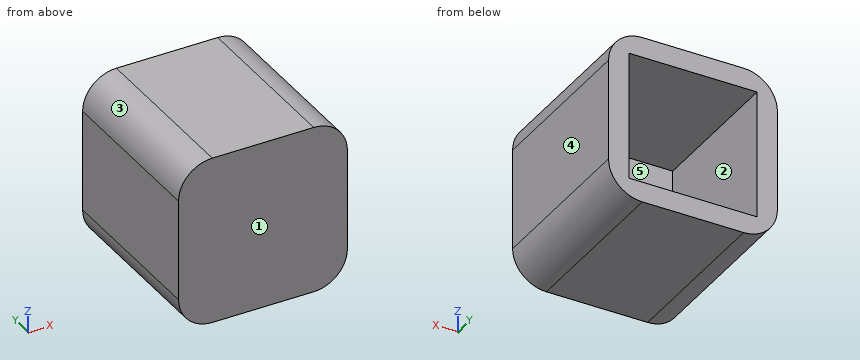
```python
from build123d import *

# Parameters (mm, degrees)
F0_W     = 25
F0_H     = 25
F1_DEPTH = 25
F2_T     = -3
F3_R     = 5
F4_R     = 5
F5_R     = 5
F6_R     = 5


with BuildPart() as f1:
    # F0 (on Top) → F1 (new body)
    with BuildSketch(Plane.XY):
        with Locations((12.5, 12.5)):
            Rectangle(F0_W, F0_H)
    extrude(amount=F1_DEPTH)

    # F2
    f2_openings = [f1.faces().sort_by_distance(p)[0] for p in [
        (12.5, 25, 12.5),
    ]]
    offset(amount=F2_T, openings=f2_openings)

    # F3
    f3_edges = [f1.edges().sort_by_distance(p)[0] for p in [
        (25, 12.5, 25),
    ]]
    fillet(f3_edges, radius=F3_R)

    # F4
    f4_edges = [f1.edges().sort_by_distance(p)[0] for p in [
        (0, 12.5, 25),
    ]]
    fillet(f4_edges, radius=F4_R)

    # F5
    f5_edges = [f1.edges().sort_by_distance(p)[0] for p in [
        (0, 12.5, 0),
    ]]
    fillet(f5_edges, radius=F5_R)

    # F6
    f6_edges = [f1.edges().sort_by_distance(p)[0] for p in [
        (25, 12.5, 0),
    ]]
    fillet(f6_edges, radius=F6_R)


solid = f1.part
```
Build history of the part. All positions in model axes, mm. Face numbers are marked on the shaded views. A direction names the side the tool comes from. Coordinates: 2 decimals unless noted, no trailing zeros. Order: outer loops, then holes, each group sorted by start corner. A loop starts at its lowest first (then second) coordinate and runs counter-clockwise, first axis right, second up. Notation, with made-up numbers: (82, 40.25) -> (141, 40.25) arc R35 ccw to (141, 74.25) -> close; hole circle Ø9 at (34.5, -40). An arc over 180 degrees is marked (long way). Answer in a Markdown table with one row per item. Add a question column.
Q1. Band-saw the part on D-D, the plane x = 2. List the corners of the cut face in (y, z), then the cut area to 3 significant figures.
Q2. Wall check: line 1 along Z through (x, y) = (9.25, 12); line 2 along Y through (x, z) = (18.75, 19). Give the ranges that are in metal, low to high. Write a range as [from, to].
Q3. Which spindle directions (+Z, -Z, +X, -X, +Y, -Y) get a long thin tool onto all of the face, cutting with end or side? Do the marked faces 4 and 5. Say none if no direction does.
Q4. Drop flat-ended pins along their axis: pin 1 (5 mm diameter, centred on x = 22, y = 10, fed in from -Z); pin 2 (8 mm diameter, centred on x = 10.5, z = 16.5, fed in from +Y). Give the stop position or say it passes through.
Q5. Band-saw the part on A-A, the plane y = 12.75. List the corners of the cut face in (x, z).
Q6. Band-saw the part on B-B, the plane x = 10.75. List the corners of the cut face in (y, z).
Q7. Band-saw the part on C-C, the plane z = 13.25. List the corners of the cut face in (x, y), then the cut area to 3 significant figures.
Q8. Mould opens along Z. For the marked faces 1, 2 and 3 say: +Z half, -Z half, draft (parallel to the pull), parting line (faces both ways), or undercut.
Answers follow:
| question | item | result |
|---|---|---|
| 1 | outline | (0, 1) -> (25, 1) -> (25, 24) -> (0, 24) -> close |
| 1 | area | 575 mm^2 |
| 2 | line 1 | [0, 3], [22, 25] |
| 2 | line 2 | [0, 3] |
| 3 | face 4 | +Z, -Z, +X, +Y, -Y |
| 3 | face 5 | +Y |
| 4 | pin 1 | z = 0 |
| 4 | pin 2 | y = 3 |
| 5 | outline | (0, 5) arc R5 ccw to (5, 0) -> (20, 0) arc R5 ccw to (25, 5) -> (25, 20) arc R5 ccw to (20, 25) -> (5, 25) arc R5 ccw to (0, 20) -> close; hole (3, 3) -> (22, 3) -> (22, 22) -> (3, 22) -> close |
| 6 | outline | (0, 0) -> (25, 0) -> (25, 3) -> (3, 3) -> (3, 22) -> (25, 22) -> (25, 25) -> (0, 25) -> close |
| 7 | outline | (0, 0) -> (25, 0) -> (25, 25) -> (22, 25) -> (22, 3) -> (3, 3) -> (3, 25) -> (0, 25) -> close |
| 7 | area | 207 mm^2 |
| 8 | face 1 | draft |
| 8 | face 2 | undercut |
| 8 | face 3 | +Z half |
